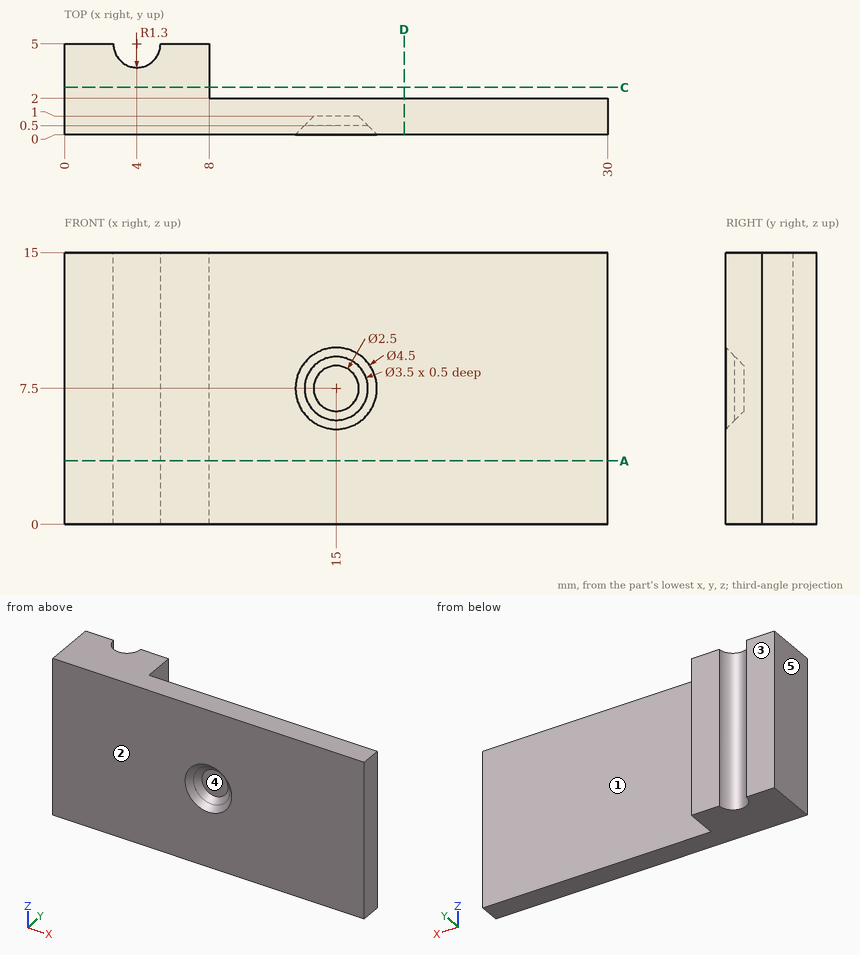
Verification items for this drawing (mm, ordinates from the low corner). A direction names the side the tool comes from. Round coordinates to 2 decimals unless told otherwise and drop trailing zeros. Loops run counter-clockwise (first coordinate to the right, second up) from the corner with the lowest first, then second, coordinate; pieces in that order, holes last. Notation, with made-up numbers: (52.25, 64.5) -> (82.25, 64.5) arc R33 ccw to (82.25, 100.5) -> close; hole circle Ø8 at (-21.5, 44). An arc over 180 degrees is marked (long way). Write item = value, one per line. Start each with the question number.
1) Sectioned sample at D-D, the plane x = 18.75. Record the cut outline in (y, z).
2) Release check for a two-part mould opening along X. For the marked faces 3, 4 and 5 record: released by +X, released by -X, zero draft, split by the parting line, or undercut.
3) Gauge pin test, flat ends, axial feed: pin 1 Ø4.5 at (x, z) = (19.5, 4) entering from +Y; pin 2 Ø3 at (x, z) = (15, 7.5) entering from -Y; pin 3 Ø2 at (y, z) = (3, 4) entering from -X; pin 4 Ø1.5 at (y, z) = (3, 10.5) entering from +X. Record the tip position at first contact, or that the pin passes through.
4) Sectioned sample at A-A, the plane z = 3.5. Record the cut outline in (x, y).
5) Thickness scan on probe 1 along X at (y, z) = (0.5, 7.5); probe 2 along Y at (x, z) = (10.5, 2.5); probe 3 along X at (y, z) = (2.4, 10.75). Record the ranges inside material, lowest first.
6) Set-up check for the marked faces 1 and 2: record each of +Z, -Z, +X, -X, +Y, -Y from which the full face is reachable in a straight line by a thin tool's end or side.
7) Sectioned sample at C-C, the plane y = 2.6. Record the cut outline in (x, z), plus the area to 3 significant figures.
Results are:
q1.outline = (0, 0) -> (2, 0) -> (2, 15) -> (0, 15) -> close
q2.face_3 = zero draft
q2.face_4 = undercut
q2.face_5 = released by -X
q3.pin_1 = 2
q3.pin_2 = 0.75
q3.pin_3 = 0
q3.pin_4 = 8
q4.outline = (0, 0) -> (30, 0) -> (30, 2) -> (8, 2) -> (8, 5) -> (5.3, 5) arc R1.3 cw to (2.7, 5) -> (0, 5) -> close
q5.probe_1 = 0 to 13.25, 16.75 to 30
q5.probe_2 = 0 to 2
q5.probe_3 = 0 to 8
q6.face_1 = +Z, -Z, +X, +Y
q6.face_2 = +Z, -Z, +X, -X, -Y
q7.outline = (0, 0) -> (8, 0) -> (8, 15) -> (0, 15) -> close
q7.area = 120 mm^2
